Source: CAD feature listing. Evaluate the final solid. Frame: model axes, mm. Face numbers are marked on the shaded views. A direction names the side the tool comes from. Round coordinates to 2 decimals unless told otherwise and drop trailing zeros. Order: outer loops, then holes, each group sorted by start corner. A loop starts at its lowest first (then second) coordinate and runs counter-clockwise, first axis right, second up. Notation, with made-up numbers: (-38.75, 48) -> (-15.75, 48) arc R11 cw to (-15.75, 57) -> close; hole circle Ø9 at (-21, -29). An arc over 180 degrees is marked (long way). One line per item, written item: value. Start each with the question number.
1) Section C-C (y = 83.5). Return the cut outline in (x, z).
2) Ray query, L1, parallel to X at y = 140.5, z = -42.5; L2, parallel to Y at x = 151.25, z = 0; L3, parallel to Y at x = -36, z = -42. Return the intervals inside material, ascending.
3) Section A-A (z = 0). Return the cut outline in (x, y), and give its area (3 significant figures).
4) Mould query, pull axis X, two halves, no side actions, for the marked faces 1, 2 and 3. Classes: pulls with the +X half, pulls with the -X half, needs draft (parallel to the pull), parting line crosses it, or undercut.
5) Reachability of the marked faces 4 and 5 from +Z, -Z, +X, -X, +Y, -Y: full face, straight path, thin tool, end or side. Return the list, or none.
6) Section B-B (y = 165). Return the cut outline in (x, z), and give its area (3 significant figures).
7) Section D-D (x = 103.5). Return the cut outline in (y, z).
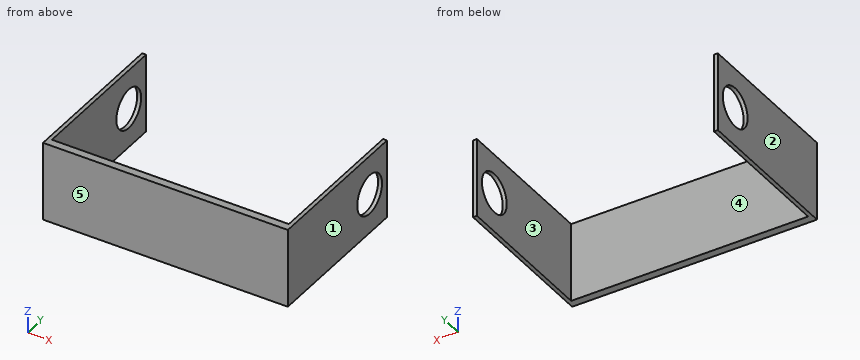
```python
from build123d import *

# Parameters (mm, degrees)
SKETCH1_W           = 300
SKETCH1_H           = 100
BOSS_EXTRUDE1_DEPTH = 10
SKETCH2_W           = 100
SKETCH2_H           = 200
BOSS_EXTRUDE2_DEPTH = 5
SKETCH3_W           = 100
SKETCH3_H           = 200
BOSS_EXTRUDE3_DEPTH = 5
CUT_EXTRUDE1_REACH  = 374.29
SKETCH4_R           = 25


with BuildPart() as part:
    # Sketch1 → Boss-Extrude1 (new body)
    with BuildSketch(Plane(origin=(0, 0, 0), x_dir=(1, 0, 0), z_dir=(0, 1, 0))):
        Rectangle(SKETCH1_W, SKETCH1_H)
    extrude(amount=BOSS_EXTRUDE1_DEPTH)

    # Sketch2 → Boss-Extrude2 (add)
    with BuildSketch(Plane(origin=(150, 0, 0), x_dir=(0, 0, -1), z_dir=(1, 0, 0))):
        with Locations((0, 100)):
            Rectangle(SKETCH2_W, SKETCH2_H)
    extrude(amount=BOSS_EXTRUDE2_DEPTH)

    # Sketch3 → Boss-Extrude3 (add)
    with BuildSketch(Plane.ZY.offset(150)):
        with Locations((0, 100)):
            Rectangle(SKETCH3_W, SKETCH3_H)
    extrude(amount=BOSS_EXTRUDE3_DEPTH)

    # Cut-Extrude1: up to this face of the body (flat: up to its plane)
    cut_extrude1_end = Plane(part.part.faces().sort_by_distance((155, 100, 0))[0])
    # Sketch4 → Cut-Extrude1 (cut, up to the picked face)
    with BuildSketch(Plane.ZY.offset(155), mode=Mode.PRIVATE) as cut_extrude1_sk1:
        with Locations((0, 165)):
            Circle(SKETCH4_R)
    cut_extrude1_tool1 = split(extrude(cut_extrude1_sk1.sketch, amount=-CUT_EXTRUDE1_REACH, mode=Mode.PRIVATE), bisect_by=cut_extrude1_end, keep=Keep.BOTH, mode=Mode.PRIVATE)
    add(cut_extrude1_tool1.solids().sort_by(Axis((-155, 165, 0), (1, 0, 0)))[0], mode=Mode.SUBTRACT)


solid = part.part
```
Findings:
1. outline: (-155, -50) -> (-150, -50) -> (-150, 50) -> (-155, 50) -> close; (150, -50) -> (155, -50) -> (155, 50) -> (150, 50) -> close
2. L1: -155 to -150, 150 to 155
2. L2: 0 to 140, 190 to 200
2. L3: 0 to 10
3. outline: (-155, 0) -> (155, 0) -> (155, 140) -> (150, 140) -> (150, 10) -> (-150, 10) -> (-150, 140) -> (-155, 140) -> close; (-155, 190) -> (-150, 190) -> (-150, 200) -> (-155, 200) -> close; (150, 190) -> (155, 190) -> (155, 200) -> (150, 200) -> close
3. area: 4,500 mm2
4. face 1: pulls with the +X half
4. face 2: pulls with the -X half
4. face 3: undercut
5. face 4: +Z, -Z, +Y
5. face 5: +Z, -Z, +X, -X, -Y
6. outline: (-155, -50) -> (-150, -50) -> (-150, -25) -> (-155, -25) -> close; (-155, 25) -> (-150, 25) -> (-150, 50) -> (-155, 50) -> close; (150, -50) -> (155, -50) -> (155, -25) -> (150, -25) -> close; (150, 25) -> (155, 25) -> (155, 50) -> (150, 50) -> close
6. area: 500 mm2
7. outline: (0, -50) -> (10, -50) -> (10, 50) -> (0, 50) -> close
